from build123d import *

# Parameters (mm, degrees)
F0_W     = 38.5
F0_H     = 50.6
F1_DEPTH = 2
F0_W_2   = 41.5
F0_H_2   = 53.6
F2_DEPTH = 21
F0_W_3   = 44.5
F0_H_3   = 56.6
F3_DEPTH = 22
F4_W     = 30.5
F4_H     = 9
F5_DEPTH = 4
F6_W     = 30.5
F6_H     = 4.5
F7_DEPTH = 4


with BuildPart() as f1:
    # F0 (on Top) → F1 (new body)
    with BuildSketch(Plane.XY):
        with Locations((-0.024678, 0.031045)):
            Rectangle(F0_W, F0_H)
    extrude(amount=F1_DEPTH)

    # F0 (on Top) → F2 (join)
    with BuildSketch(Plane.XY):
        with Locations((-0.024678, 0.031045)):
            Rectangle(F0_W_2, F0_H_2)
        with Locations((-0.024678, 0.031045)):
            Rectangle(F0_W, F0_H, mode=Mode.SUBTRACT)
    extrude(amount=F2_DEPTH)

    # F0 (on Top) → F3 (join)
    with BuildSketch(Plane.XY):
        with Locations((-0.024678, 0.031045)):
            Rectangle(F0_W_3, F0_H_3)
        with Locations((-0.024678, 0.031045)):
            Rectangle(F0_W_2, F0_H_2, mode=Mode.SUBTRACT)
    extrude(amount=F3_DEPTH)

    # F4 (on face) → F5 (cut)
    with BuildSketch(Plane(origin=(0, 28.331045, 0), x_dir=(-1, 0, 0), z_dir=(0, 1, 0))):
        with Locations((0.024678, 17.5)):
            Rectangle(F4_W, F4_H)
    extrude(amount=-F5_DEPTH, mode=Mode.SUBTRACT)

    # F6 (on face) → F7 (cut)
    with BuildSketch(Plane.XY):
        with Locations((-0.024678, -22.018955)):
            Rectangle(F6_W, F6_H)
    extrude(amount=F7_DEPTH, mode=Mode.SUBTRACT)


solid = f1.part
Part model, mm, in its own coordinate system. A direction names the side the tool comes from. Give positions to 0.01 mm unless a question says otherwise; leave off trailing zeros. Order: outer loops, then holes, each group sorted by start corner. A loop starts at its lowest first (then second) coordinate and runs counter-clockwise, first axis right, second up. Notation, with made-up numbers: (9.5, 77) - (18.5, 77) arc R12 cw to (18.5, 93) - close; hole circle Ø10 at (-10.75, 81.5). An arc over 180 degrees is marked (long way). One line per question, with ' | ' between items.
1. Which spindle directions (+Z, -Z, +X, -X, +Y, -Y) get a long thin tool onto all of the face, cutting with end or side? Do faces 4 (the face through (-15.275, 27, 17)), 5 (the face through (0, 28.331, 8)), 6 (the face through (0, 0, 0)), 7 (the face through (-19.275, 0, 11)), 8 (the face through (0, -24.269, 1)). Say none if no direction does.
Filled in:
face 4: +Z, +Y | face 5: +Z, -Z, +X, -X, +Y | face 6: -Z, +X, -X, +Y, -Y | face 7: +Z | face 8: +Z, -Z
2. Pull direction X, two halves, no side cores. Call faces 1 (the face through (0, -27, 22)), 2 (the face through (-20, -6, 21)), 3 (the face through (22.225, 0, 11)): +X half, -X half, draft (parallel to the pull), parting line (faces both ways), or undercut.
Filled in:
face 1: draft | face 2: undercut | face 3: +X half
3. Drill centre lines: probe 1 along X at (y, z) = (24, 2.25); probe 2 along Y at (x, z) = (-19, 3.5); probe 3 along Y at (x, z) = (-12, 18.5). Where is each one in solid material? Low to high.
Filled in:
probe 1: -22.27 to -19.27, 19.23 to 22.23 | probe 2: -28.27 to -25.27, 25.33 to 28.33 | probe 3: -28.27 to -25.27
4. Band-saw the part on D-D on x = 18.5. List the corners of the cut face in (y, z), then the cut area to 3 significant figures.
Filled in:
outline: (-28.27, 0) - (28.33, 0) - (28.33, 22) - (26.83, 22) - (26.83, 21) - (25.33, 21) - (25.33, 2) - (-25.27, 2) - (-25.27, 21) - (-26.77, 21) - (-26.77, 22) - (-28.27, 22) - close | area: 230 mm²
5. Band-saw the part on B-B on x = 3. List the corners of the cut face in (y, z).
Filled in:
outline: (-28.27, 0) - (-24.27, 0) - (-24.27, 2) - (-25.27, 2) - (-25.27, 21) - (-26.77, 21) - (-26.77, 22) - (-28.27, 22) - close; (-19.77, 0) - (28.33, 0) - (28.33, 13) - (25.33, 13) - (25.33, 2) - (-19.77, 2) - close
6. Band-saw the part on C-C on z = 19.5. List the corners of the cut face in (x, y).
Filled in:
outline: (-22.27, -28.27) - (22.23, -28.27) - (22.23, 28.33) - (15.23, 28.33) - (15.23, 25.33) - (19.23, 25.33) - (19.23, -25.27) - (-19.27, -25.27) - (-19.27, 25.33) - (-15.27, 25.33) - (-15.27, 28.33) - (-22.27, 28.33) - close
7. Drop flat-ended pins along their axis: P1, Ø12, axis at x = -10, y = 18.5, coming from the +Z side; P2, Ø3, axis at x = 2, z = 17.5, coming from the +Y side; P3, Ø2.5, axis at x = -3, y = 26.5, coming from the +Z side. Give the stop position or say it passes through.
Filled in:
P1: z = 2 | P2: y = -25.27 | P3: z = 13
8. Band-saw the part on A-A on y = -23.5. List the corners of the cut face in (x, z).
Filled in:
outline: (-22.27, 0) - (-15.27, 0) - (-15.27, 2) - (-19.27, 2) - (-19.27, 21) - (-20.77, 21) - (-20.77, 22) - (-22.27, 22) - close; (15.23, 0) - (22.23, 0) - (22.23, 22) - (20.73, 22) - (20.73, 21) - (19.23, 21) - (19.23, 2) - (15.23, 2) - close
